Source: CAD feature listing. Evaluate the final solid. Frame: model axes, mm. A direction names the side the tool comes from. Give positions to 0.01 mm unless a question says otherwise; leave off trailing zeros. Order: outer loops, then holes, each group sorted by start corner. A loop starts at its lowest first (then second) coordinate and runs counter-clockwise, first axis right, second up. Notation, with made-up numbers: (61, 0.25) - (68, 0.25) arc R21 ccw to (68, 5.25) - close; hole circle Ø4 at (36.5, 28.25). An arc over 180 degrees is marked (long way). Use CSV: the item, a comma, the result in double quotes.
```python
from build123d import *

# Parameters (mm, degrees)
SALIENTE_EXTRUIR1_DEPTH      = 6.35
TALADRO_DE_MARGEN_PARA_M41_D = 4.5
REDONDEO1_R                  = 5


# Read off the part's stored shape, not the designer's step: Saliente-Extruir1
with BuildPart() as part:
    # Saliente-Extruir1 outline → Saliente-Extruir1 (new body)
    with BuildSketch(Plane(origin=(0, 0, 0), x_dir=(0, 0, -1), z_dir=(1, 0, 0))):
        with BuildLine():
            Line((-2.5, 180), (-17.5, 180))
            Line((-17.5, 180), (-17.5, 100))
            add(Edge.make_bspline(
                [(-17.5, 100), (-17.5, 98.712751966), (-17.500047788, 96.116321069), (-17.51148981, 91.098940131), (-17.565479393, 85.046877218), (-17.737925717, 78.203948852), (-18.147729277, 69.656133307), (-19.038911227, 60.095322328), (-20.718334539, 50.310614009), (-22.956153632, 41.771686415), (-25.785586207, 33.773608765), (-29.338865081, 25.548124026), (-33.697565336, 16.449967912), (-38.713561507, 6.016494532), (-43.953609584, -6.016361906), (-48.809754323, -19.661313126), (-52.733015331, -34.671033487), (-55.439087369, -50.654463146), (-56.694005293, -64.452671708), (-57.222054598, -75.565918854), (-57.428472519, -83.87427142), (-57.487938926, -90.701655992), (-57.499988878, -96.070691027), (-57.5, -98.684323127), (-57.5, -100)],
                knots=[0, 0, 0, 0, 0.015625, 0.03125, 0.0625, 0.09375, 0.125, 0.1875, 0.25, 0.3125, 0.375, 0.4375, 0.5, 0.5625, 0.625, 0.6875, 0.75, 0.8125, 0.875, 0.90625, 0.9375, 0.96875, 0.984375, 1, 1, 1, 1], degree=3))
            Line((-57.5, -100), (-57.5, -180))
            Line((-57.5, -180), (-42.5, -180))
            Line((-42.5, -180), (-42.5, -150))
            Line((-42.5, -150), (2.5, -150))
            Line((2.5, -150), (2.5, -180))
            Line((2.5, -180), (17.5, -180))
            Line((17.5, -180), (17.5, -100))
            add(Edge.make_bspline(
                [(17.5, -100), (17.5, -98.712751966), (17.500047788, -96.116321069), (17.51148981, -91.098940131), (17.565479393, -85.046877218), (17.737925717, -78.203948852), (18.147729277, -69.656133307), (19.038911227, -60.095322328), (20.718334539, -50.310614009), (22.956153632, -41.771686415), (25.785586207, -33.773608765), (29.338865081, -25.548124026), (33.697565336, -16.449967912), (38.713561507, -6.016494532), (43.953609584, 6.016361906), (48.809754323, 19.661313126), (52.733015331, 34.671033487), (55.439087369, 50.654463146), (56.694005293, 64.452671708), (57.222054598, 75.565918854), (57.428472519, 83.87427142), (57.487938926, 90.701655992), (57.499988878, 96.070691027), (57.5, 98.684323127), (57.5, 100)],
                knots=[0, 0, 0, 0, 0.015625, 0.03125, 0.0625, 0.09375, 0.125, 0.1875, 0.25, 0.3125, 0.375, 0.4375, 0.5, 0.5625, 0.625, 0.6875, 0.75, 0.8125, 0.875, 0.90625, 0.9375, 0.96875, 0.984375, 1, 1, 1, 1], degree=3))
            Line((57.5, 100), (57.5, 180))
            Line((57.5, 180), (42.5, 180))
            Line((42.5, 180), (42.5, 60))
            Line((42.5, 60), (-2.5, 60))
            Line((-2.5, 60), (-2.5, 180))
        make_face()
    extrude(amount=SALIENTE_EXTRUIR1_DEPTH)

    # Taladro de margen para M41 (through all)
    with Locations(Plane.ZY):
        with Locations((10, 163), (10, 175), (-50, 163), (-50, 175), (50, -175), (50, -163), (-10, -175), (-10, -163)):
            Hole(TALADRO_DE_MARGEN_PARA_M41_D / 2)

    # Redondeo1
    redondeo1_edges = [part.edges().sort_by_distance(p)[0] for p in [
        (3.175, 180, 2.5),
        (3.175, 180, -42.5),
        (3.175, 180, -57.5),
        (3.175, -180, -17.5),
        (3.175, -180, -2.5),
        (3.175, -180, 42.5),
        (3.175, -180, 57.5),
        (3.175, 180, 17.5),
    ]]
    fillet(redondeo1_edges, radius=REDONDEO1_R)


solid = part.part
```
Item 1: Material intervals for line 1 (Z direction, x = 4, y = -175); line 2 (Y direction, x = 4, z = -10); line 3 (Y direction, x = 4.25, z = 10), sorted ascending. Write a range as from..to.
Filled in:
line 1,"z = -17.5..-12.25, -7.75..-2.5, 42.5..47.75, 52.25..57.5"
line 2,"y = -180..-177.25, -172.75..-165.25, -160.75..60"
line 3,"y = -150..160.75, 165.25..172.75, 177.25..180"
Item 2: First-contact query: pin 1 (3 mm diameter, centred on x = 4, y = 155.5, fed in from +Z); pin 2 (3 mm diameter, centred on x = 4, y = -142, fed in from -Z); pin 3 (2 mm diameter, centred on x = 5, z = 14.5, fed in from +Y). Flat tips, straight axial feed; report the tip coordinate or a pass-through.
Filled in:
pin 1,"stops at z = 17.5"
pin 2,"stops at z = -17.5"
pin 3,"stops at y = 179.9"
Item 3: Section B-B on x = 1.25. Count the separate pieces of the cut face and the enclosed holes in it, then the cut area to 3 significant figures.
Filled in:
separate pieces,"1"
enclosed holes,"8"
area,"20,600 mm2"
Item 4: Mould query, pull axis Z, two halves, no side actions, for faces 1 (the flat face through (0, -37, 1)), 2 (the flat face through (3, -163, 42.5)), 3 (the flat face through (3, -137, 57.5)), 4 (the flat face through (3, 137, -57.5)). Classes: released by +Z, released by -Z, zero draft, split by the parting line, or undercut.
Filled in:
face 1,"zero draft"
face 2,"undercut"
face 3,"released by +Z"
face 4,"released by -Z"
Item 5: Section A-A on y = -113. Return the cut outline in (x, z), then the cut area to 3 significant figures.
Filled in:
outline,"(0, -17.5) - (6.35, -17.5) - (6.35, 57.5) - (0, 57.5) - close"
area,"476 mm2"
Item 6: Set-up query: faces 5 (the flat face through (3, 138, 17.5)), 6 (the flat face through (6.35, -37, 1)), 7 (the flat face through (3, -138, -17.5)), 8 (the flat face through (3, 117, 2.5)), 9 (the flat face through (3, -150, 20)). Return all of +Z, -Z, +X, -X, +Y, -Y with unobstructed straight access to the full face (end or side cutting, diameter ignored); none if empty.
Filled in:
face 5,"+Z, +X, -X, +Y"
face 6,"+Z, -Z, +X, +Y, -Y"
face 7,"-Z, +X, -X, -Y"
face 8,"+X, -X, +Y"
face 9,"+X, -X, -Y"
